Geometry check sheet. Reference: the model listing, model coordinates, mm. A direction names the side the tool comes from. Give positions to 0.01 mm unless a question says otherwise; leave off trailing zeros. Write each loop counter-clockwise with the first axis right and the second up, starting at its lowest first coordinate (ties: lowest second). Pieces come first, ordered by that corner, then holes.
(1) Cross-section at A-A (y = 42.5). Record the boundary of the cut face in (x, z).
(2) Cross-section at B-B (z = 21.5). Record the boundary of the cut face in (x, y).
(3) Depth check by flat-ended pin: P1, Ø1.5, axis at y = 15, z = 2, coming from the -X side; P2, Ø4.5, axis at x = 42, y = 69, coming from the -Z side; P3, Ø2, axis at x = -1.5, y = -47.5, coming from the -Z side; P4, Ø3, axis at x = 0, y = 42.5, coming from the -Z side. Enter the tip coordinate at first touch or a pass-through.
(4) Cross-section at C-C (x = -28). Record the boundary of the cut face in (y, z), and give its area (3 significant figures).
(5) Mould release check, pull along Z, two halves, no side actions. Record for faces 4 (the flat face through (0, -75, 45.8)), 5 (the cylindrical face through (0.63, -76.07, 53.5)), 6 (the cylindrical face through (-48.57, -76, 27.82)): +Z half, -Z half, draft (parallel to the pull), parting line (faces both ways), or undercut.
(6) Cross-section at D-D (z = 8). Record the boundary of the cut face in (x, y).
(7) Tool access check on faces 1 (the flat face through (42, 70, 11.5)), 2 (the cylindrical face through (-1.517, -34.334, 52.535)), 3 (the flat face through (-8, -74, 48.8)). Record the directions out of +Z, -Z, +X, -X, +Y, -Y that give a thin tool (end or side, any length) a straight path to the whole face; none if there is none.
(8) Thickness scan on line 1 along Y through (x, z) = (-15.5, 41); line 2 along X through (y, z) = (-45, 17.5); line 3 along Y through (x, z) = (0, 51). Record the ranges inside material, lowest first.
```python
from build123d import *

# Parameters (mm, degrees)
SKETCH6_W           = 100
SKETCH6_H           = 155
BOSS_EXTRUDE5_DEPTH = 55
FILLET2_R           = 5
SHELL3_START        = -45
SHELL3_OUTLINE_W    = 145
SHELL3_OUTLINE_H    = 50
SHELL3_DEPTH        = 90
BOSS_EXTRUDE6_DEPTH = 45
SKETCH8_R           = 2.1
CUT_EXTRUDE1_DEPTH  = 6.5
SKETCH9_R           = 2.5
SKETCH9_R_2         = 3
SKETCH9_R_3         = 7
CUT_EXTRUDE2_DEPTH  = 108.383657975
CUT_EXTRUDE3_REACH  = 173.901
CUT_EXTRUDE4_START  = -3
CUT_EXTRUDE4_DEPTH  = 3
BOSS_EXTRUDE7_DEPTH = 3
SKETCH15_W          = 90.6
SKETCH15_H          = 145.6
CUT_EXTRUDE5_DEPTH  = 5


# Read off the part's stored shape, not the designer's step: Shell3
with BuildPart() as part:
    # Sketch6 → Boss-Extrude5 (new body)
    with BuildSketch(Plane.XY):
        Rectangle(SKETCH6_W, SKETCH6_H)
    extrude(amount=BOSS_EXTRUDE5_DEPTH)

    # Fillet2
    fillet2_edges = [part.edges().sort_by_distance(p)[0] for p in [
        (-50, 0, 55),
        (0, -77.5, 55),
        (50, 0, 55),
        (0, -77.5, 0),
        (-50, 0, 0),
        (0, 77.5, 0),
        (50, 0, 0),
        (50, -77.5, 27.5),
        (-50, -77.5, 27.5),
        (-50, 77.5, 27.5),
        (50, 77.5, 27.5),
        (0, 77.5, 55),
    ]]
    fillet(fillet2_edges, radius=FILLET2_R)

    # Shell3 outline → Shell3 (cut)
    with BuildSketch(Plane.YZ.offset(SHELL3_START)):
        with Locations((0, 25)):
            Rectangle(SHELL3_OUTLINE_W, SHELL3_OUTLINE_H)
    extrude(amount=SHELL3_DEPTH, mode=Mode.SUBTRACT)

    # Sketch7 → Boss-Extrude6 (add)
    with BuildSketch(Plane(origin=(0, 0, 50), x_dir=(-1, 0, 0), z_dir=(0, 0, -1))):
        with BuildLine():
            Line((-45, 72.5), (-37, 72.5))
            Line((-37, 72.5), (-37, 71.5))
            ThreePointArc((-37, 71.5), (-39.050252532, 66.550252532), (-44, 64.5))
            Line((-44, 64.5), (-45, 64.5))
            Line((-45, 64.5), (-45, 72.5))
        make_face()
        with BuildLine():
            Line((45, 72.5), (37, 72.5))
            Line((37, 72.5), (37, 71.5))
            ThreePointArc((37, 71.5), (39.050252532, 66.550252532), (44, 64.5))
            Line((44, 64.5), (45, 64.5))
            Line((45, 64.5), (45, 72.5))
        make_face()
        with BuildLine():
            Line((-45, -64.5), (-44, -64.5))
            ThreePointArc((-44, -64.5), (-39.050252532, -66.550252532), (-37, -71.5))
            Line((-37, -71.5), (-37, -72.5))
            Line((-37, -72.5), (-45, -72.5))
            Line((-45, -72.5), (-45, -64.5))
        make_face()
        with BuildLine():
            Line((45, -72.5), (45, -64.5))
            Line((45, -64.5), (44, -64.5))
            ThreePointArc((44, -64.5), (39.050252532, -66.550252532), (37, -71.5))
            Line((37, -71.5), (37, -72.5))
            Line((37, -72.5), (45, -72.5))
        make_face()
    extrude(amount=BOSS_EXTRUDE6_DEPTH)

    # Sketch8 → Cut-Extrude1 (cut)
    with BuildSketch(Plane(origin=(0, 0, 5), x_dir=(-1, 0, 0), z_dir=(0, 0, -1))):
        with Locations((-42, 69.5)):
            Circle(SKETCH8_R)
        with Locations((42, 69.5)):
            Circle(SKETCH8_R)
        with Locations((42, -69.5)):
            Circle(SKETCH8_R)
        with Locations((-42, -69.5)):
            Circle(SKETCH8_R)
    extrude(amount=-CUT_EXTRUDE1_DEPTH, mode=Mode.SUBTRACT)

    # Sketch9 → Cut-Extrude2 (cut, through all)
    with BuildSketch(Plane.XY.offset(55)):
        with Locations((0, 42.5)):
            Circle(SKETCH9_R)
        with Locations((0, 7.5)):
            Circle(SKETCH9_R_2)
        with Locations((0, -27.5)):
            Circle(SKETCH9_R_3)
    extrude(amount=-CUT_EXTRUDE2_DEPTH, mode=Mode.SUBTRACT)

    # Sketch10 → Cut-Extrude3 (cut, up to next)
    with BuildSketch(Plane.XZ.offset(77.5), mode=Mode.PRIVATE) as cut_extrude3_sk1:
        with BuildLine():
            Line((-3.5, 50), (3.5, 50))
            ThreePointArc((3.5, 50), (4.914213562, 49.414213562), (5.5, 48))
            Line((5.5, 48), (5.5, 47.8))
            ThreePointArc((5.5, 47.8), (4.914213562, 46.385786438), (3.5, 45.8))
            Line((3.5, 45.8), (-3.5, 45.8))
            ThreePointArc((-3.5, 45.8), (-4.914213562, 46.385786438), (-5.5, 47.8))
            Line((-5.5, 47.8), (-5.5, 48))
            ThreePointArc((-5.5, 48), (-4.914213562, 49.414213562), (-3.5, 50))
        make_face()
    cut_extrude3_tool1 = extrude(cut_extrude3_sk1.sketch, amount=-CUT_EXTRUDE3_REACH, mode=Mode.PRIVATE) & part.part
    add(cut_extrude3_tool1.solids().sort_by_distance((0, -77.5, 47.9))[0], mode=Mode.SUBTRACT)

    # Sketch13 → Cut-Extrude4 (cut)
    with BuildSketch(Plane(origin=(0, -72.5, 0), x_dir=(1, 0, 0), z_dir=(0, 1, 0)).offset(CUT_EXTRUDE4_START)):
        with BuildLine():
            Line((5.5, -47.8), (5.5, -48))
            ThreePointArc((5.5, -48), (5.457812626, -48.408619287), (5.333030278, -48.8))
            Line((5.333030278, -48.8), (10.333030278, -48.8))
            Line((10.333030278, -48.8), (10.333030278, -50))
            Line((10.333030278, -50), (3.5, -50))
            Line((3.5, -50), (-3.5, -50))
            Line((-3.5, -50), (-10.333030278, -50))
            Line((-10.333030278, -50), (-10.333030278, -48.8))
            Line((-10.333030278, -48.8), (-5.333030278, -48.8))
            ThreePointArc((-5.333030278, -48.8), (-5.457812626, -48.408619287), (-5.5, -48))
            Line((-5.5, -48), (-5.5, -47.8))
            ThreePointArc((-5.5, -47.8), (-4.914213562, -46.385786438), (-3.5, -45.8))
            Line((-3.5, -45.8), (3.5, -45.8))
            ThreePointArc((3.5, -45.8), (4.914213562, -46.385786438), (5.5, -47.8))
        make_face()
    extrude(amount=CUT_EXTRUDE4_DEPTH, mode=Mode.SUBTRACT)

    # Sketch14 → Boss-Extrude7 (add)
    with BuildSketch(Plane(origin=(0, 0, 50), x_dir=(-1, 0, 0), z_dir=(0, 0, -1))):
        with BuildLine():
            Line((-7.5, -46.6), (7.5, -46.5))
            Line((7.5, -46.5), (7.5, -46.6))
            ThreePointArc((7.5, -46.6), (6.943502884, -47.943502884), (5.6, -48.5))
            Line((5.6, -48.5), (-5.6, -48.5))
            ThreePointArc((-5.6, -48.5), (-6.943502884, -47.943502884), (-7.5, -46.6))
        make_face()
    extrude(amount=BOSS_EXTRUDE7_DEPTH)

    # Sketch15 → Cut-Extrude5 (cut)
    with BuildSketch(Plane(origin=(0, 0, 0), x_dir=(-1, 0, 0), z_dir=(0, 0, -1))):
        Rectangle(SKETCH15_W, SKETCH15_H)
    extrude(amount=-CUT_EXTRUDE5_DEPTH, mode=Mode.SUBTRACT)


solid = part.part
```
Reply:
1. outline: (-50, 5) arc R5 ccw to (-45.3, 0.01) - (-45.3, 5) - (-45, 5) - (-45, 50) - (-2.5, 50) - (-2.5, 55) - (-45, 55) arc R5 ccw to (-50, 50) - close; (2.5, 50) - (45, 50) - (45, 5) - (45.3, 5) - (45.3, 0.01) arc R5 ccw to (50, 5) - (50, 50) arc R5 ccw to (45, 55) - (2.5, 55) - close
2. outline: (-50, -72.5) arc R5 ccw to (-45, -77.5) - (45, -77.5) arc R5 ccw to (50, -72.5) - (50, 72.5) arc R5 ccw to (45, 77.5) - (-45, 77.5) arc R5 ccw to (-50, 72.5) - close; hole (-45, -64.5) - (-44, -64.5) arc R7 cw to (-37, -71.5) - (-37, -72.5) - (37, -72.5) - (37, -71.5) arc R7 cw to (44, -64.5) - (45, -64.5) - (45, 64.5) - (44, 64.5) arc R7 cw to (37, 71.5) - (37, 72.5) - (-37, 72.5) - (-37, 71.5) arc R7 cw to (-44, 64.5) - (-45, 64.5) - close
3. P1: stops at x = -49.47
3. P2: stops at z = 5
3. P3: stops at z = 47
3. P4: passes through
4. outline: (-77.5, 5) arc R5 ccw to (-72.8, 0.01) - (-72.8, 5) - (-72.5, 5) - (-72.5, 50) - (72.5, 50) - (72.5, 5) - (72.8, 5) - (72.8, 0.01) arc R5 ccw to (77.5, 5) - (77.5, 50) arc R5 ccw to (72.5, 55) - (-72.5, 55) arc R5 ccw to (-77.5, 50) - close
4. area: 1,250 mm2
5. face 4: undercut
5. face 5: +Z half
5. face 6: draft
6. outline: (-50, -72.5) arc R5 ccw to (-45, -77.5) - (45, -77.5) arc R5 ccw to (50, -72.5) - (50, 72.5) arc R5 ccw to (45, 77.5) - (-45, 77.5) arc R5 ccw to (-50, 72.5) - close; hole (-45, -64.5) - (-44, -64.5) arc R7 cw to (-37, -71.5) - (-37, -72.5) - (37, -72.5) - (37, -71.5) arc R7 cw to (44, -64.5) - (45, -64.5) - (45, 64.5) - (44, 64.5) arc R7 cw to (37, 71.5) - (37, 72.5) - (-37, 72.5) - (-37, 71.5) arc R7 cw to (-44, 64.5) - (-45, 64.5) - close; hole circle Ø4.2 at (-42, -69.5); hole circle Ø4.2 at (-42, 69.5); hole circle Ø4.2 at (42, -69.5); hole circle Ø4.2 at (42, 69.5)
7. face 1: -Z
7. face 2: +Z, -Z
7. face 3: none
8. line 1: y = -77.5 to -72.5, 72.5 to 77.5
8. line 2: x = -50 to -45, 45 to 50
8. line 3: y = -77.4 to -34.5, -20.5 to 4.5, 10.5 to 40, 45 to 77.4
